Can you work these out from the drawing? Everything is in mm from the part's minimum corner. Round coordinates to 2 decimals unless told otherwise and drop trailing zeros. Loops run counter-clockwise (first coordinate to the right, second up) from the corner with the lowest first, then second, coordinate; pieces in that order, holes last. Notation, with made-up numbers: (11, 38) -> (38, 38) arc R23 cw to (38, 46) -> close; hole circle Ø1 at (-35.75, 23.25). An arc over 180 degrees is marked (long way). One line per item, written item: value.
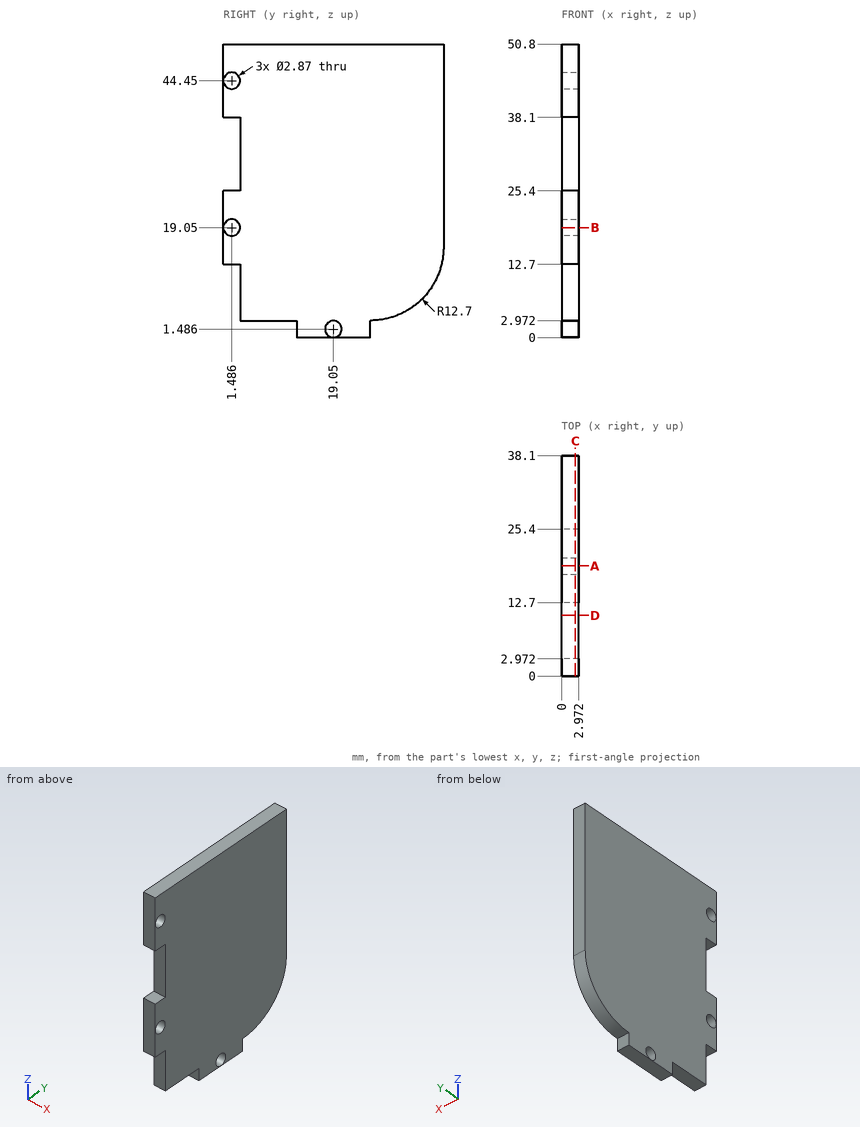
(1) If we section it at D-D, the plane y = 10.5: Please give me the cut outline in (x, z), then the cut area to 3 significant figures.
Recorded:
outline: (0, 2.97) -> (2.97, 2.97) -> (2.97, 50.8) -> (0, 50.8) -> close
area: 142 mm²
(2) If I drill on L1, parallel to Y at x = 1.65, z = 33; L2, parallel to Z at x = 1.3, y = 18.5; L3, parallel to Z at x = 0.3, y = 20, over which ranges is the centre line in solid material (lowest first)?
Recorded:
L1: 2.97 to 38.1
L2: 0 to 0.16, 2.81 to 50.8
L3: 0 to 0.41, 2.56 to 50.8
(3) I'm going to push flat-ended pins straight in: pin 1 Ø1.5 at (x, z) = (1, 30.5) entering from -Y; pin 2 Ø1.5 at (x, z) = (1, 2) entering from +Y; pin 3 Ø1.5 at (x, y) = (2, 1.5) entering from -Z. Where does each tip first touch, or does it pass through?
Recorded:
pin 1: y = 2.97
pin 2: y = 25.4
pin 3: z = 12.7
(4) If we section it at A-A, the plane y = 19.05: Please give me the cut outline in (x, z).
Recorded:
outline: (0, 0) -> (2.97, 0) -> (2.97, 0.05) -> (0, 0.05) -> close; (0, 2.92) -> (2.97, 2.92) -> (2.97, 50.8) -> (0, 50.8) -> close
(5) If we section it at B-B, the plane z = 19.05: Please give me the cut outline in (x, y).
Recorded:
outline: (0, 0) -> (2.97, 0) -> (2.97, 0.05) -> (0, 0.05) -> close; (0, 2.92) -> (2.97, 2.92) -> (2.97, 38.1) -> (0, 38.1) -> close
(6) If we section it at C-C, the plane x = 2.4: Give the number of separate pieces and of enclosed holes in the cut face, then the cut area to 3 significant figures.
Recorded:
separate pieces: 1
enclosed holes: 3
area: 1,740 mm²
